Could you check a few things on this drawing? It's one solid part, dimensions in mm from its lowest x, y, z. A direction names the side the tool comes from. Give positions to 0.01 mm unless a question says otherwise; leave off trailing zeros. Loops run counter-clockwise (first coordinate to the right, second up) from the corner with the lowest first, then second, coordinate; pieces in that order, holes last. Notation, with made-up numbers: (42.25, 48.25) - (57.25, 48.25) arc R19 cw to (57.25, 79.25) - close; hole circle Ø11 at (50, -16.75). An arc over 180 degrees is marked (long way). Return JSON: item names as keys, results as strings. Group by question number.
(1) If we section it at A-A (y = 2): Please give me the cut outline in (x, z), then the cut area to 3 significant figures.
(2) On a 3-axis mill with a long thin cutter (end or side, diameter ignored), from which of +Z, -Z, +X, -X, +Y, -Y can I reach the whole of each face in a straight line? I mean the marked faces 1 and 2. Say none if no direction works.
(3) I need wall thicknesses on probe 1 along Z at (x, y) = (1.4, 3.5); probe 2 along Z at (x, y) = (2.15, 5.5); probe 3 along Y at (x, z) = (2.85, 7). Which ranges of each line are inside material? Lowest first, please. Write a range as [from, to].
(4) For P1, Ø1.3, axis at x = 3, y = 5, coming from the +Z side; P2, Ø4, axis at y = 6.5, z = 5.5, coming from the -X side, each with a flat end and sliding along its axis, tell me the tip position at first contact or that it passes through.
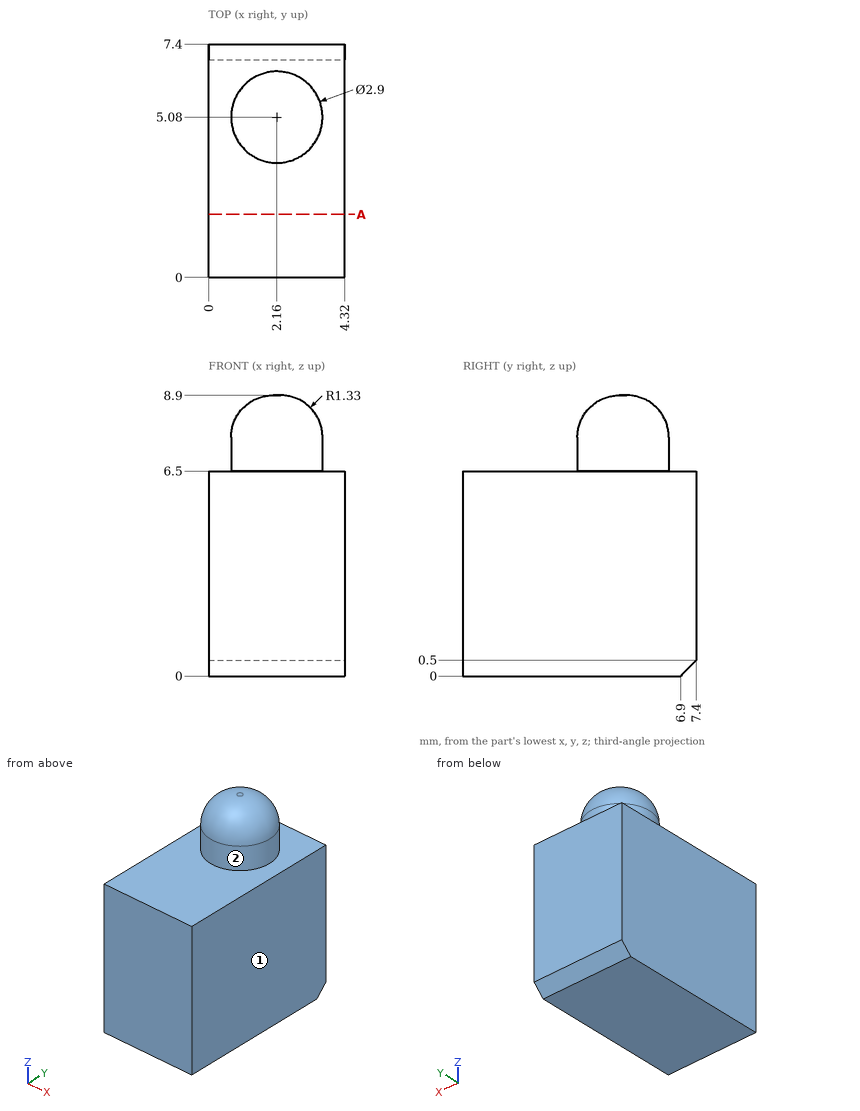
Values:
{
 "1": {"outline": "(0, 0) - (4.32, 0) - (4.32, 6.5) - (0, 6.5) - close", "area": "28.1 mm2"},
 "2": {"face 1": "+Z, -Z, +X, +Y, -Y", "face 2": "+Z"},
 "3": {"probe 1": "[0, 6.5]", "probe 2": "[0, 8.87]", "probe 3": "[3.8, 6.36]"},
 "4": {"P1": "z = 8.9", "P2": "x = 0"}
}
